```python
from build123d import *

# Parameters (mm, degrees)
F0_R     = 1.2
F1_DEPTH = 3.5


with BuildPart() as f1:
    # F0 (on Top) → F1 (new body)
    with BuildSketch(Plane.XY):
        Polygon((20, -5), (10, 5), (0, 5), (-10, -5), align=None)
        with Locations((-1.093396, -2.093396)):
            Circle(F0_R, mode=Mode.SUBTRACT)
        with Locations((11.093396, -2.093396)):
            Circle(F0_R, mode=Mode.SUBTRACT)
    extrude(amount=F1_DEPTH)


with BuildPart() as f2_1:
    # F2: copy of F1
    add(f1.part)


solid = f2_1.part
```
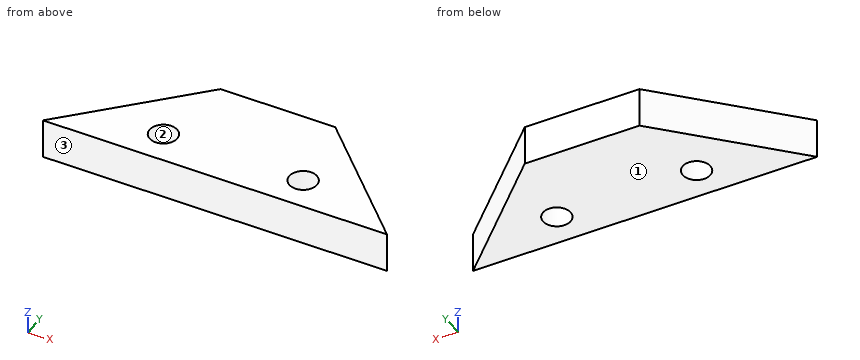
The model under review builds one solid part; all positions refer to its coordinate system, in mm. Face numbers are marked on the shaded views. Coordinates: 2 decimals unless noted, no trailing zeros. Loops run counter-clockwise (first coordinate to the right, second up) from the corner with the lowest first, then second, coordinate; pieces in that order, holes last. Notation, with made-up numbers: (18, 17) -> (50, 17) arc R25 cw to (50, 56) -> close; hole circle Ø5 at (89.5, -14). An arc over 180 degrees is marked (long way). Answer as CSV lines item,"result".
Item 1: Take a section at C-C, the plane z = 0.9. State the section outline as (x, y) points, and give its area (3 significant figures).
Results below:
outline,"(-10, -5) -> (20, -5) -> (10, 5) -> (0, 5) -> close; hole circle Ø2.4 at (-1.09, -2.09); hole circle Ø2.4 at (11.09, -2.09)"
area,"191 mm2"
Item 2: Insertion check: pin 1 (1.5 mm diameter, centred on y = -2.5, z = 1.5, fed in from +X); pin 2 (1 mm diameter, centred on y = 2.5, z = 2, fed in from -X). Each pin has a flat end and moves straight along its axis. Give the tip position at first contact, or say it passes through.
Results below:
pin 1,"stops at x = 18.25"
pin 2,"stops at x = -3"
Item 3: Take a section at D-D, the plane x = 17.75. State the section outline as (y, z) points, and give its area (4 significant figures).
Results below:
outline,"(-5, 0) -> (-2.75, 0) -> (-2.75, 3.5) -> (-5, 3.5) -> close"
area,"7.875 mm2"
Item 4: Take a section at B-B, the plane y = -3. State the section outline as (x, z) points.
Results below:
outline,"(-8, 0) -> (-1.88, 0) -> (-1.88, 3.5) -> (-8, 3.5) -> close; (-0.31, 0) -> (10.31, 0) -> (10.31, 3.5) -> (-0.31, 3.5) -> close; (11.88, 0) -> (18, 0) -> (18, 3.5) -> (11.88, 3.5) -> close"
Item 5: Take a section at A-A, the plane x = 10.75. State the section outline as (y, z) points.
Results below:
outline,"(-5, 0) -> (-3.24, 0) -> (-3.24, 3.5) -> (-5, 3.5) -> close; (-0.94, 0) -> (4.25, 0) -> (4.25, 3.5) -> (-0.94, 3.5) -> close"
Item 6: For L1, parallel to X at y = -1.75, z = 2.9; L2, parallel to X at y = -2.25, z = 0.9; L3, parallel to Y at x = -1.25, z = 2.6, list the stretches that pass through material, from the lowest coordinate up.
Results below:
L1,"x = -6.75 to -2.24, 0.06 to 9.94, 12.24 to 16.75"
L2,"x = -7.25 to -2.28, 0.1 to 9.9, 12.28 to 17.25"
L3,"y = -5 to -3.28, -0.9 to 3.75"
Item 7: Draft analysis for pull direction Y (two halves, no side actions). For the marked faces 1, 2 and 3, state which applies: +Y half, -Y half, draft (parallel to the pull), parting line (faces both ways), or undercut.
Results below:
face 1,"draft"
face 2,"undercut"
face 3,"-Y half"
